Can you work these out from the model? Positions are in its coordinate system, mm. Face numbers are marked on the shaded views. A direction names the side the tool comes from. Give positions to 0.01 mm unless a question says otherwise; leave off trailing zeros. Order: outer loops, then holes, each group sorted by start corner. A loop starts at its lowest first (then second) coordinate and runs counter-clockwise, first axis right, second up. Notation, with made-up numbers: M -3.75,46.25 L 13.25,46.25 A27 cw 13.25,84.25 Z; hole C 45.5,-9.5 d2. An arc over 180 degrees is marked long. Use one line per item in the form item = value. Start each with the question number.
1. For the marked faces 1 and 2, which set-ups out of +Z, -Z, +X, -X, +Y, -Y let a thin tool reach every point of the face, with its end or its side?
2. I want a section at B-B, the plane z = 5. List the corners of the cut face in (x, y) for me, and give its area (3 significant figures).
3. I want a section at A-A, the plane y = 18. List the corners of the cut face in (x, z) for me.
4. I need wall thicknesses on L1, parallel to Z at x = 40, y = 12.5; L2, parallel to X at y = 30.5, z = 5; L3, parallel to X at y = 30.5, z = 3. Which ranges of each line are inside material? Lowest first, please.
5. I want a section at C-C, the plane z = 8.25. List the corners of the cut face in (x, y) for me.
6. Will this pin go through, and if not, where does the flat tip stop? P1, Ø5, axis at y = 24.5, z = 3, coming from the -X side.
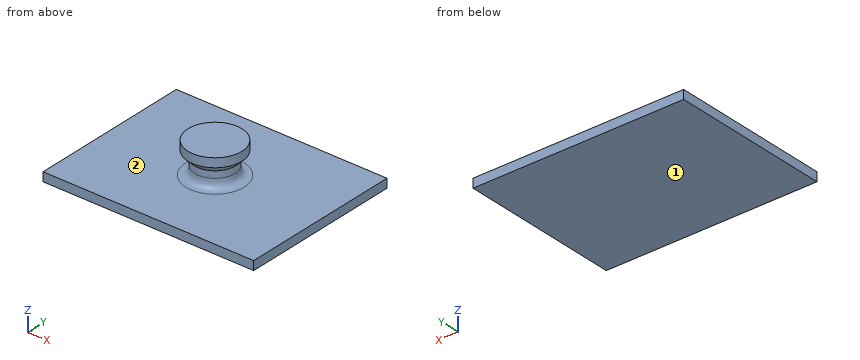
```python
from build123d import *

# Parameters (mm, degrees)
SKETCH1_W           = 47
SKETCH1_H           = 36
BOSS_EXTRUDE1_DEPTH = 2
SKETCH2_R           = 4.5
BOSS_EXTRUDE2_DEPTH = 5
SKETCH3_R           = 6
BOSS_EXTRUDE3_DEPTH = 2
FILLET1_SIZE        = 2
CHAMFER1_SIZE       = 1.5


# Some blends are built 0.0001 mm under size
with BuildPart() as part:
    # Sketch1 → Boss-Extrude1 (new body)
    with BuildSketch(Plane.XY):
        with Locations((23.5, 28.347826087)):
            Rectangle(SKETCH1_W, SKETCH1_H)
    extrude(amount=BOSS_EXTRUDE1_DEPTH)

    # Sketch2 → Boss-Extrude2 (add)
    with BuildSketch(Plane.XY.offset(2)):
        with Locations((23.5, 28.347826087)):
            Circle(SKETCH2_R)
    extrude(amount=BOSS_EXTRUDE2_DEPTH)

    # Sketch3 → Boss-Extrude3 (add)
    with BuildSketch(Plane.XY.offset(7)):
        with Locations((23.5, 28.347826087)):
            Circle(SKETCH3_R)
    extrude(amount=BOSS_EXTRUDE3_DEPTH)

    # Fillet1
    # a fillet whose section is not a circle: 2 mm, written as the material it adds along each edge
    with BuildSketch(Plane(origin=(23.5, 28.347826087, 2), x_dir=(1, 0, 0), z_dir=(0, -1, 0))) as fillet1_piece_1:
        with BuildLine():
            add(Edge.make_bspline([(4.5, FILLET1_SIZE), (4.5, FILLET1_SIZE * 0.831801948466), (4.5, FILLET1_SIZE * 0.663603896932), (4.5 + FILLET1_SIZE * 0.0716919198361, FILLET1_SIZE * 0.292893218813), (4.5 + FILLET1_SIZE * 0.292893218813, FILLET1_SIZE * 0.0716919198361), (4.5 + FILLET1_SIZE * 0.663603896932, 0), (4.5 + FILLET1_SIZE * 0.831801948466, 0), (4.5 + FILLET1_SIZE, 0)], knots=[0, 0, 0, 0, 0, 0, 0.5, 0.5, 1, 1, 1, 1, 1, 1], degree=5))
            Line((4.5 + FILLET1_SIZE, 0), (4.5, 0))
            Line((4.5, 0), (4.5, FILLET1_SIZE))
        make_face()
    revolve(axis=Axis((23.5, 28.347826087, 2), (0, 0, 1)))

    # Chamfer1
    chamfer1_edges = [part.edges().sort_by_distance(p)[0] for p in [
        (19, 28.347826087, 7),
    ]]
    chamfer(chamfer1_edges, length=CHAMFER1_SIZE - 0.0001)  # a hair under: the kernel refuses the full size


solid = part.part
```
Check result:
q1.face_1 = -Z, +X, -X, +Y, -Y
q1.face_2 = +Z
q2.outline = C 23.5,28.35 d9
q2.area = 63.6 mm2
q3.outline = M 0,0 L 47,0 L 47,2 L 0,2 Z
q4.L1 = 0 to 2
q4.L2 = 19.55 to 27.45
q4.L3 = 19.42 to 27.58
q5.outline = C 23.5,28.35 d12
q6.P1 = 0
